Autodesk Inventor part; units mm, degrees
ref_plane "YZ Plane" through (0, 0, 0) normal (1, 0, 0) x (0, 1, 0)
ref_plane "XZ Plane" through (0, 0, 0) normal (0, 1, 0) x (-1, 0, 0)
ref_plane "XY Plane" through (0, 0, 0) normal (0, 0, 1) x (1, 0, 0)
sketch "Sketch1" plane through (0, 0, 0) normal (0, 1, 0) x (-1, 0, 0)
  line L0 (0, 0) -> (0, -411.151) construction
  line L1 (-4, 0) -> (-4, -411.151)
  line L2 (4, -411.151) -> (4, 0)
  arc A0 (4, 0) -> (-4, 0) centre (0, 0) ccw
  arc A1 (-4, -411.151) -> (4, -411.151) centre (0, -411.151) ccw
  circle A2 centre (0, -411.151) radius 1.5
  circle A3 centre (0, 0) radius 1.5
  circle A4 centre (0, -77.048) radius 1.5
  point P0 (0, -205.5755)
  dimension "d0" = 411.151
  dimension "d1" = 8
  dimension "d2" = 3
  dimension "d3" = 3
  dimension "d6" = 3
  dimension "d7" = 334.103
extrude "Extrusion1" add sketch "Sketch1" along normal blind 4.5
sketch "Sketch2" plane through (0, 4.5, 0) normal (0, 1, 0) x (1, 0, 0)
  arc A0 (4, 411.151) -> (-4, 411.151) centre (0, 411.151) ccw
  line L0 (-4, 411.151) -> (-4, 0)
  arc A1 (-4, 0) -> (4, 0) centre (0, 0) ccw
  line L1 (4, 0) -> (4, 411.151)
  circle A2 centre (0, 77.048) radius 1.5
  circle A3 centre (0, 0) radius 1.5
  circle A4 centre (0, 411.151) radius 1.5
properties part number "Wing_arm_2"
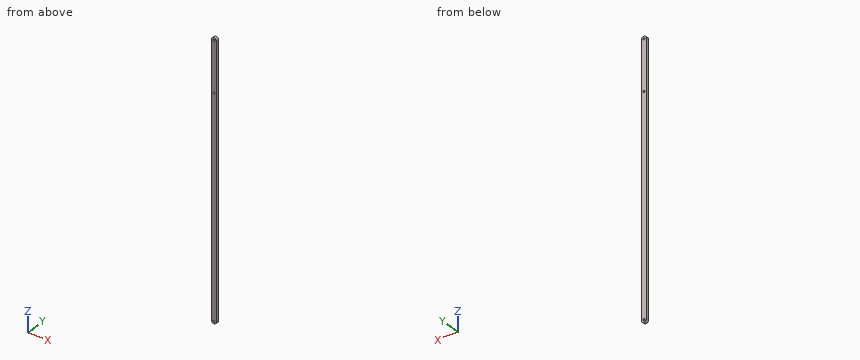
The listing builds one solid part. Answer for the finished solid, in the listing's coordinates (mm). Round coordinates to 2 decimals unless told otherwise and drop trailing zeros. Write each loop counter-clockwise with the first axis right and the second up, starting at its lowest first coordinate (ties: lowest second). Pieces come first, ordered by that corner, then holes. Notation, with made-up numbers: (-4, 6.25) - (43, 6.25) arc R9 cw to (43, 10.25) - close; hole circle Ø1 at (41, -18.5). An arc over 180 degrees is marked (long way). Use one line per item in the form item = value. Start each with the question number.
Item 1: Find the intervals of material crossed by line 1 (Z direction, x = 0, y = 2.9); line 2 (Z direction, x = 0.25, y = 2.7); line 3 (Z direction, x = -2.5, y = 2.5), in increasing order. Write a range as [from, to].
Item 2: Flat-ended cylindrical pins translate along their axes: pin 1 Ø1.5 at (x, y) = (1, 0.5) entering from -Z; pin 2 Ø1.5 at (x, y) = (-2, 1.5) entering from -Z. Find the tip coordinate at first contact, or state that the pin passes through.
Item 3: A cutting plane is placed at A-A (x = 0). Write down the section's boundary in (y, z), plus the area to 3 significant figures.
The answers:
q1.line_1 = [-415.15, -412.65], [-409.65, -78.55], [-75.55, -1.5], [1.5, 4]
q1.line_2 = [-415.14, -412.63], [-409.67, -78.53], [-75.57, -1.48], [1.48, 3.99]
q1.line_3 = [-414.27, 3.12]
q2.pin_1 = -415.14
q2.pin_2 = -414.95
q3.outline = (0, -415.15) - (4.5, -415.15) - (4.5, -412.65) - (0, -412.65) - close; (0, -409.65) - (4.5, -409.65) - (4.5, -78.55) - (0, -78.55) - close; (0, -75.55) - (4.5, -75.55) - (4.5, -1.5) - (0, -1.5) - close; (0, 1.5) - (4.5, 1.5) - (4.5, 4) - (0, 4) - close
q3.area = 1,850 mm^2
